Could you check a few things on this model? Use its own coordinates, in mm. A direction names the side the tool comes from. Give positions to 0.01 mm unless a question says otherwise; leave off trailing zeros. Write each loop counter-clockwise with the first axis right and the second up, starting at its lowest first coordinate (ties: lowest second). Pieces come first, ordered by that corner, then holes. Notation, with made-up numbers: M -30,-14.5 L 4,-14.5 A15 ccw 4,8.5 Z; hole C 50,34.25 d7. An arc over 180 degrees is marked long. Answer as a JSON object with one key per item and string values. Group by question number.
Autodesk Inventor part; units mm, degrees
ref_plane "YZ Plane" through (0, 0, 0) normal (1, 0, 0) x (0, 1, 0)
ref_plane "XZ Plane" through (0, 0, 0) normal (0, 1, 0) x (-1, 0, 0)
ref_plane "XY Plane" through (0, 0, 0) normal (0, 0, 1) x (1, 0, 0)
sketch "Sketch1" plane through (0, 0, 0) normal (0, 0, 1) x (1, 0, 0)
  line L0 (0, 278.716) -> (197.082, 197.082) construction
  line L1 (197.082, 197.082) -> (278.716, 0) construction
  line L2 (278.716, 0) -> (197.082, -197.082) construction
  line L3 (197.082, -197.082) -> (0, -278.716) construction
  line L4 (0, -278.716) -> (-197.082, -197.082) construction
  line L5 (-197.082, -197.082) -> (-278.716, 0) construction
  line L6 (-278.716, 0) -> (-197.082, 197.082) construction
  line L7 (-197.082, 197.082) -> (0, 278.716)
  line L8 (-197.082, 197.082) -> (0, 278.716)
  line L9 (-461.6493, 774.8136) -> (-221.4406, 874.3113)
  line L10 (-98.541, 237.899) -> (-341.545, 824.5625) construction
  line L11 (-221.4406, 874.3113) -> (0, 874.3113)
  line L12 (0, 874.3113) -> (0, 278.716)
  line L13 (-461.6493, 774.8136) -> (-618.2315, 618.2315)
  line L14 (-618.2315, 618.2315) -> (-197.082, 197.082)
  point P0 (0, 0)
  point P1 (0, 0)
  dimension "d0" = 515
  dimension "d2" = 260
  dimension "d3" = 635
extrude "Extrusion1" add sketch "Sketch1" along normal mid plane 8
sketch "Sketch2" plane through (0, 0, 4) normal (0, 0, 1) x (1, 0, 0)
  line L0 (-221.4406, 874.3113) -> (-461.6493, 774.8136)
  line L1 (-461.6493, 774.8136) -> (-618.2315, 618.2315)
  line L2 (-236.7713, 532.4196) -> (-415.8262, 458.2526)
  line L3 (-197.082, 197.082) -> (0, 278.716)
  line L4 (-98.541, 237.899) -> (-341.545, 824.5625) construction
  line L5 (-618.2315, 618.2315) -> (-197.082, 197.082)
  line L6 (-415.8262, 458.2526) -> (-575.8051, 618.2315)
  line L7 (-575.8051, 618.2315) -> (-444.6557, 749.3809)
  line L8 (-444.6557, 749.3809) -> (-343.9227, 791.1058)
  line L9 (-236.7713, 532.4196) -> (-343.9227, 791.1058)
  line L10 (-209.0549, 543.9001) -> (-30, 618.067)
  line L11 (-30, 618.067) -> (-30, 844.3113)
  line L12 (-30, 844.3113) -> (-215.4733, 844.3113)
  line L13 (-215.4733, 844.3113) -> (-316.2063, 802.5863)
  line L14 (-209.0549, 543.9001) -> (-316.2063, 802.5863)
  line L15 (0, 278.716) -> (0, 874.3113)
  line L16 (-415.8262, 458.2526) -> (-30, 618.067) construction
  line L17 (-392.8652, 435.2916) -> (-30, 585.5953)
  line L18 (-190.043, 232.4694) -> (-30, 298.7614)
  line L19 (-30, 298.7614) -> (-30, 585.5953)
  line L20 (-190.043, 232.4694) -> (-392.8652, 435.2916)
  point P0 (0, 0)
  dimension "d11" = 30
  dimension "d12" = 280
  dimension "d13" = 30
  dimension "d14" = 30
  dimension "d15" = 15
  dimension "d21" = 30
  dimension "d22" = 30
  dimension "d23" = 30
  dimension "d24" = 30
extrude "Extrusion2" cut sketch "Sketch2" against normal up to surface (8 mm away)
fillet "Fillet1" radius 10 12 edges at (-575.8051, 618.2315, 0) (-343.9227, 791.1058, 0) (-236.7713, 532.4196, 0) (-415.8262, 458.2526, 0) (-316.2063, 802.5863, 0) (-30, 844.3113, 0) (-30, 618.067, 0) (-209.0549, 543.9001, 0) (-392.8652, 435.2916, 0) (-30, 585.5953, 0) (-30, 298.7614, 0) (-190.043, 232.4694, 0)
sketch "Sketch5" plane through (0, 0, 4) normal (0, 0, 1) x (1, 0, 0)
  line L0 (-221.4406, 874.3113) -> (-461.6493, 774.8136)
  line L1 (0, 874.3113) -> (-221.4406, 874.3113)
  line L2 (-461.6493, 774.8136) -> (-618.2315, 618.2315)
  line L3 (-618.2315, 618.2315) -> (-197.082, 197.082)
  line L4 (-197.082, 197.082) -> (0, 278.716)
  line L5 (0, 278.716) -> (0, 874.3113)
  line L6 (-15, 859.3113) -> (-218.4569, 859.3113) construction
  line L7 (-218.4569, 859.3113) -> (-453.1525, 762.0973) construction
  line L8 (-453.1525, 762.0973) -> (-597.0183, 618.2315) construction
  line L9 (-597.0183, 618.2315) -> (-193.5625, 214.7757) construction
  line L10 (-193.5625, 214.7757) -> (-15, 288.7387) construction
  line L11 (-15, 288.7387) -> (-15, 859.3113) construction
  line L12 (-379.0384, 441.0189) -> (-43.8268, 579.868)
  line L13 (-212.8817, 553.1389) -> (-312.3794, 793.3476)
  line L14 (-419.3457, 440.5589) -> (-15, 608.0444) construction
  line L15 (-217.1728, 524.3016) -> (-335.8047, 810.7043) construction
  circle A0 centre (-335.8047, 810.7043) radius 2
  circle A1 centre (-217.1728, 524.3016) radius 2
  circle A2 centre (-296.262, 715.2398) radius 2
  circle A3 centre (-256.7194, 619.7753) radius 2
  circle A4 centre (-597.0183, 618.2315) radius 2
  circle A5 centre (-516.2262, 537.4394) radius 2
  circle A6 centre (-435.4342, 456.6474) radius 2
  circle A7 centre (-354.6421, 375.8553) radius 2
  circle A8 centre (-273.8501, 295.0633) radius 2
  circle A9 centre (-193.0581, 214.2713) radius 2
  circle A10 centre (-317.4138, 482.7805) radius 2
  circle A11 centre (-104.2812, 251.7572) radius 2
  circle A12 centre (-519.2365, 696.0132) radius 2
  circle A13 centre (-437.4315, 768.6091) radius 2
  circle A14 centre (-15, 859.3113) radius 2
  circle A15 centre (-15, 745.0541) radius 2
  circle A16 centre (-15, 630.7969) radius 2
  circle A17 centre (-15, 516.5397) radius 2
  circle A18 centre (-15, 402.2825) radius 2
  circle A19 centre (-15, 288.0253) radius 2
  circle A20 centre (-116.9319, 565.8228) radius 2
  circle A21 centre (-125, 859.3113) radius 2
  circle A22 centre (-234.178, 852.7995) radius 2
  point P0 (0, 0)
  dimension "d32" = 15
  dimension "d33" = 15
  dimension "d34" = 15
  dimension "d35" = 4
  dimension "d37" = 103.33
  dimension "d38" = 103.33
  dimension "d43" = 114.2572
  dimension "d49" = 108.5
  dimension "d50" = 110
  dimension "d51" = 110
extrude "Extrusion4" cut sketch "Sketch5" against normal up to surface (8 mm away) contours A0 | A1 | A2 | A3 | A4 | A5 | A6 | A7 | A8 | A9 | A10 | A11 | A12 | A13 | A14 | A15 | A16 | A17 | A18 | A19 | A20 | A21 | A22
equation "\"d0\" = Барабан_размер_по_плоскостям"
equation "\"d2\" = Кассета_длина_грани"
equation "\"d3\" = Кассета_высота"
equation "\"d11\" = d13"
equation "\"d14\" = d13"
equation "\"d15\" = 0.5 * d13"
equation "\"d21\" = d13"
equation "\"d22\" = d13"
equation "\"d23\" = d13"
equation "\"d24\" = d13"
properties part number "DMF 01 56 Крепление сетки к кассете v2.1"
1) Please list where these lines run through material, in increasing order: line 1 along X through (y, z) = (712, -3); line 2 along Y through (x, z) = (-92.5, -0.25); line 3 along X through (y, z) = (629.5, 2.5). Write a range as from..to.
2) For faces 5 (the flat face through (-213.78, 509.47, 0.06)), 6 (the flat face through (-99.921, 237.328, -0.056)), which set-ups out of +Z, -Z, +X, -X, +Y, -Y let a thin tool reach every point of the face, with its end or its side?
3) If we section it at B-B, the plane x = -502: List the corners of the cut face in (y, z) for me.
4) If we section it at C-C, the plane y = 600: List the corners of the cut face in (x, z) for me, plus the area to 3 significant figures.
5) I'm going to push flat-ended pins straight in: pin 1 (2 mm diameter, centred on x = -291.5, z = 1, fed in from +Y); pin 2 (2 mm diameter, centred on x = -211.5, z = -2.5, fed in from -Y); pin 3 (4 mm diameter, centred on x = -430.5, z = 3, fed in from +Y). Where does each tip first touch, or does it pass through?
6) If we section it at D-D, the plane x = -61: List the corners of the cut face in (y, z) for me.
7) We'd pull the mould along Y, two halves only. Please class faces 1 (the flat face through (-538.844, 697.619, -0.056)), 2 (the flat face through (-261.934, 671.562, 0.056)), 3 (the flat face through (-119.14, 581.144, 0.056)), 4 (the flat face through (-242, 562, -4)): released by +Y, released by -Y, zero draft, split by the parting line, or undercut.
8) If we section it at A-A, the plane y = 271: List the corners of the cut face in (x, z) for me.
Taken from the geometry:
{
 "1": {"line 1": "-524.46..-482.04, -311.16..-278.68, -30..0", "line 2": "240.4..272.87, 559.71..592.18, 844.31..874.31", "line 3": "-606.96..-564.54, -276.98..-244.51, -30..-16.52, -13.48..0"},
 "2": {"face 5": "+Z, -Z", "face 6": "+Z, -Z, +X, -Y"},
 "3": {"outline": "M 502,-4 L 544.43,-4 L 544.43,4 L 502,4 Z; M 692.04,-4 L 734.46,-4 L 734.46,4 L 692.04,4 Z"},
 "4": {"outline": "M -600,-4 L -557.57,-4 L -557.57,4 L -600,4 Z; M -264.76,-4 L -232.29,-4 L -232.29,4 L -264.76,4 Z; M -73.62,-4 L 0,-4 L 0,4 L -73.62,4 Z", "area": "1,190 mm²"},
 "5": {"pin 1": "y = 845.71", "pin 2": "y = 210.5", "pin 3": "y = 788.54"},
 "6": {"outline": "M 253.45,-4 L 285.92,-4 L 285.92,4 L 253.45,4 Z; M 572.75,-4 L 605.23,-4 L 605.23,4 L 572.75,4 Z; M 844.31,-4 L 874.31,-4 L 874.31,4 L 844.31,4 Z"},
 "7": {"face 1": "released by +Y", "face 2": "undercut", "face 3": "undercut", "face 4": "zero draft"},
 "8": {"outline": "M -271,-4 L -228.57,-4 L -228.57,4 L -271,4 Z; M -97.02,-4 L -18.63,-4 L -18.63,4 L -97.02,4 Z"}
}
